```python
from build123d import *

# Parameters (mm, degrees)
BASE_EXTRUDE_DEPTH = 5


with BuildPart() as part:
    # Sketch1 → Base-Extrude (new body)
    with BuildSketch(Plane.XY):
        with BuildLine():
            Line((-90, 97), (-90, 65.232555285))
            ThreePointArc((-90, 65.232555285), (-87.704928127, 56.437372938), (-81.404974165, 49.885032327))
            Line((-81.404974165, 49.885032327), (-12.531200021, 7.679129249))
            ThreePointArc((-12.531200021, 7.679129249), (-10.560110304, 7.264321725), (-8.770963462, 8.189639794))
            ThreePointArc((-8.770963462, 8.189639794), (0, 12), (8.770963462, 8.189639794))
            ThreePointArc((8.770963462, 8.189639794), (10.560110304, 7.264321725), (12.531200021, 7.679129249))
            Line((12.531200021, 7.679129249), (81.404974165, 49.885032327))
            ThreePointArc((81.404974165, 49.885032327), (87.704928127, 56.437372938), (90, 65.232555285))
            Line((90, 65.232555285), (90, 97))
            ThreePointArc((90, 97), (89.121320344, 99.121320344), (87, 100))
            Line((87, 100), (80.100622615, 100))
            ThreePointArc((80.100622615, 100), (78.379893306, 99.457456133), (77.281544752, 98.02606043))
            Line((77.281544752, 98.02606043), (74.969567775, 91.67395589))
            ThreePointArc((74.969567775, 91.67395589), (70.816403532, 83.984822172), (64.623472754, 77.818854371))
            Line((64.623472754, 77.818854371), (17.844683603, 43.204371262))
            ThreePointArc((17.844683603, 43.204371262), (0, 37.320077081), (-17.844683603, 43.204371262))
            Line((-17.844683603, 43.204371262), (-64.623472754, 77.818854371))
            ThreePointArc((-64.623472754, 77.818854371), (-70.816403532, 83.984822172), (-74.969567775, 91.67395589))
            Line((-74.969567775, 91.67395589), (-77.281544752, 98.02606043))
            ThreePointArc((-77.281544752, 98.02606043), (-78.379893306, 99.457456133), (-80.100622615, 100))
            Line((-80.100622615, 100), (-87, 100))
            ThreePointArc((-87, 100), (-89.121320344, 99.121320344), (-90, 97))
        make_face()
    extrude(amount=BASE_EXTRUDE_DEPTH)


solid = part.part
```
Could you check a few things on this model? Use its own coordinates, in mm. A direction names the side the tool comes from. Give positions to 0.01 mm unless a question says otherwise; leave off trailing zeros. Loops run counter-clockwise (first coordinate to the right, second up) from the corner with the lowest first, then second, coordinate; pieces in that order, holes last. Notation, with made-up numbers: (63, 10) - (110, 10) arc R10 ccw to (110, 21) - close; hole circle Ø5 at (-24, 22.25). An arc over 180 degrees is marked (long way). Answer in a Markdown table with one row per item. Add a question column.
Q1. For pin 1 (1 mm diameter, centred on y = 43, z = 1, fed in from -X); pin 2 (3 mm diameter, centred on x = 3.5, z = 4, fed in from +Y); pin 3 (3 mm diameter, centred on x = -42, z = 1, fed in from +Y), each with a flat end and sliding along its axis, tell me the tip position at first contact or that it passes through.
Q2. If we section it at D-D (x = -1): List the corners of the cut face in (y, z) for me, plus the area to 3 significant figures.
Q3. If we section it at B-B (z = 0.9): List the corners of the cut face in (x, y) for me.
Q4. If we section it at C-C (y = 87): List the corners of the cut face in (x, z) for me.
Q5. We'd pull the mould along X, two halves only. Please class faces 1 (the face through (90, 81, 2)), 2 (the face through (70.9, 84.1, 2.5)), 3 (the face through (-1, 34, 5)), 4 (the face through (-40.91, 60.27, 2.46)): +X half, -X half, draft (parallel to the pull), parting line (faces both ways), or undercut.
Q6. Please list where these lines run through material, in increasing order: L1, parallel to X at y = 49, z = 3.75; L2, parallel to Y at x = 20.5, z = 2.1; L3, parallel to Y at x = -38.5, z = 2.65. Write a range as from..to.
Q7. If we section it at A-A (y = 63.5): List the corners of the cut face in (x, z) for me, plus the area to 3 significant figures.
Q8. Which directions (+Z, -Z, +X, -X, +Y, -Y) give clear straight access to the entire face, cutting with the end or side of a thin tool? Please do faces 5 (the face through (-1, 34, 0)), 6 (the face through (76.14, 94.89, 2.46)).
The answers:
| question | item | result |
|---|---|---|
| 1 | pin 1 | stops at x = -70.99 |
| 1 | pin 2 | stops at y = 37.74 |
| 1 | pin 3 | stops at y = 62.19 |
| 2 | outline | (11.96, 0) - (37.34, 0) - (37.34, 5) - (11.96, 5) - close |
| 2 | area | 127 mm^2 |
| 3 | outline | (-90, 65.23) arc R18 ccw to (-81.4, 49.89) - (-12.53, 7.68) arc R3 ccw to (-8.77, 8.19) arc R12 cw to (8.77, 8.19) arc R3 ccw to (12.53, 7.68) - (81.4, 49.89) arc R18 ccw to (90, 65.23) - (90, 97) arc R3 ccw to (87, 100) - (80.1, 100) arc R3 ccw to (77.28, 98.03) - (74.97, 91.67) arc R30 cw to (64.62, 77.82) - (17.84, 43.2) arc R30 cw to (-17.84, 43.2) - (-64.62, 77.82) arc R30 cw to (-74.97, 91.67) - (-77.28, 98.03) arc R3 ccw to (-80.1, 100) - (-87, 100) arc R3 ccw to (-90, 97) - close |
| 4 | outline | (-90, 0) - (-72.8, 0) - (-72.8, 5) - (-90, 5) - close; (72.8, 0) - (90, 0) - (90, 5) - (72.8, 5) - close |
| 5 | face 1 | +X half |
| 5 | face 2 | undercut |
| 5 | face 3 | draft |
| 5 | face 4 | undercut |
| 6 | L1 | x = -79.96..-25.68, 25.68..79.96 |
| 6 | L2 | y = 12.56..45.17 |
| 6 | L3 | y = 23.59..58.49 |
| 7 | outline | (-89.92, 0) - (-45.27, 0) - (-45.27, 5) - (-89.92, 5) - close; (45.27, 0) - (89.92, 0) - (89.92, 5) - (45.27, 5) - close |
| 7 | area | 446 mm^2 |
| 8 | face 5 | -Z, +X, -X, +Y, -Y |
| 8 | face 6 | +Z, -Z, +Y |
